from build123d import *

# Parameters (mm, degrees)
F0_W     = 13
F0_H     = 5
F1_DEPTH = 12
F2_W     = 11.2
F2_H     = 2
F3_DEPTH = 12
F4_W     = 9.4
F4_H     = 2
F5_DEPTH = 5.001
F7_DEPTH = 13
F8_W     = 1
F8_H     = 4
F9_DEPTH = 13.001


with BuildPart() as f1:
    # F0 (on Top) → F1 (new body)
    with BuildSketch(Plane.XY):
        Rectangle(F0_W, F0_H)
    extrude(amount=F1_DEPTH)

    # F2 (on face) → F3 (cut)
    with BuildSketch(Plane.XY.offset(12)):
        with Locations((0, 0.6)):
            Rectangle(F2_W, F2_H)
    extrude(amount=-F3_DEPTH, mode=Mode.SUBTRACT)

    # F4 (on face) → F5 (cut, through all)
    with BuildSketch(Plane(origin=(0, 2.5, 0), x_dir=(-1, 0, 0), z_dir=(0, 1, 0))):
        with Locations((0, 6)):
            Rectangle(F4_W, F4_H)
    extrude(amount=-F5_DEPTH, mode=Mode.SUBTRACT)

    # F6 (on face) → F7 (join)
    with BuildSketch(Plane(origin=(-6.5, 0, 0), x_dir=(0, -1, 0), z_dir=(-1, 0, 0))):
        with BuildLine():
            ThreePointArc((4.472136, -9.454356), (5.605034, -7.595289), (6, -5.454356))
            ThreePointArc((6, -5.454356), (5.049752, -2.213986), (2.5, 0))
            Line((2.5, 0), (-2.5, 0))
            ThreePointArc((-2.5, 0), (-5.873575, -4.229155), (-4.472136, -9.454356))
            ThreePointArc((-4.472136, -9.454356), (-1.428948, -1.652564), (5.25, -6.704356))
            ThreePointArc((5.25, -6.704356), (5.051792, -8.133304), (4.472136, -9.454356))
        make_face()
    extrude(amount=-F7_DEPTH)

    # F8 (on face) → F9 (cut, through all)
    with BuildSketch(Plane(origin=(-6.5, 0, 0), x_dir=(0, -1, 0), z_dir=(-1, 0, 0))):
        with Locations((0, 0.52178)):
            Rectangle(F8_W, F8_H)
    extrude(amount=-F9_DEPTH, mode=Mode.SUBTRACT)


solid = f1.part
Verification items for the finished model (mm, model axes). A direction names the side the tool comes from. Give positions to 0.01 mm unless a question says otherwise; leave off trailing zeros. Write each loop counter-clockwise with the first axis right and the second up, starting at its lowest first coordinate (ties: lowest second). Pieces come first, ordered by that corner, then holes. Notation, with made-up numbers: M 9,53 L 35,53 A26 cw 35,77 Z; hole C -38.75,62.25 d1. An arc over 180 degrees is marked long. Put each result on its own line as item: value. Start each with the question number.
1. Scan lines: line 1 along Y through (x, z) = (-5.5, 11.25); line 2 along X through (y, z) = (-0.5, 6.75); line 3 along X through (y, z) = (1.25, 5.25). Record each from-to range of solid material in increasing order. Write a range as [from, to].
2. Draft check along Z on faces 1 (the face through (5.6, 1, 6)), 2 (the face through (0, -1, 12)), 3 (the face through (0, -1, 5)). Enter one of: +Z half, -Z half, draft (parallel to the pull), parting line (faces both ways), or undercut.
3. Section check A-A (y = 0). Record the cut outline in (x, z).
4. Section check D-D (z = 8.75). Record the cut outline in (x, y), and give its area (3 significant figures).
5. Set-up check for faces 4 (the face through (-0.1, 0.5, -0.4)), 5 (the face through (-5.6, 1, 6)), 6 (the face through (-0.1, -0.4, 7.3)), 7 (the face through (4.7, 2, 6)), 8 (the face through (-0.09, 4.73, -4.43)): record each of +Z, -Z, +X, -X, +Y, -Y from which the full face is reachable in a straight line by a thin tool's end or side.
6. Go/stop test with flat-tipped pins: pin 1 Ø2 at (x, z) = (-0.5, -0.5) entering from -Y; pin 2 Ø5.5 at (x, z) = (-0.5, 4.5) entering from -Y; pin 3 Ø0.6 at (x, y) = (0.5, -1.5) entering from -Z. Record where each tip stops, or that it passes through.
7. Section check B-B (z = 6.5). Record the cut outline in (x, y).
8. Section check C-C (x = 2). Record the cut outline in (y, z), and give its area (3 significant figures).
Answer list:
1. line 1: [-2.5, -0.4], [1.6, 2.5]
1. line 2: [-6.5, -4.7], [4.7, 6.5]
1. line 3: [-6.5, -5.6], [5.6, 6.5]
2. face 1: draft
2. face 2: +Z half
2. face 3: undercut
3. outline: M -6.5,2.52 L -5.6,2.52 L -5.6,12 L -6.5,12 Z; M 5.6,2.52 L 6.5,2.52 L 6.5,12 L 5.6,12 Z
4. outline: M -6.5,-2.5 L 6.5,-2.5 L 6.5,2.5 L -6.5,2.5 Z; hole M -5.6,-0.4 L 5.6,-0.4 L 5.6,1.6 L -5.6,1.6 Z
4. area: 42.6 mm2
5. face 4: -Z, +X, -X
5. face 5: +Z
5. face 6: +Z, -Z
5. face 7: +Y, -Y
5. face 8: +X, -X
6. pin 1: y = -4.51
6. pin 2: y = -2.5
6. pin 3: z = -1.77
7. outline: M -6.5,-2.5 L -4.7,-2.5 L -4.7,-0.4 L -5.6,-0.4 L -5.6,1.6 L -4.7,1.6 L -4.7,2.5 L -6.5,2.5 Z; M 4.7,-2.5 L 6.5,-2.5 L 6.5,2.5 L 4.7,2.5 L 4.7,1.6 L 5.6,1.6 L 5.6,-0.4 L 4.7,-0.4 Z
8. outline: M -6,-5.45 A6 ccw -4.47,-9.45 A5.25 cw -5.25,-6.7 A5.25 cw -0.5,-1.48 L -0.5,2.52 L -0.4,2.52 L -0.4,5 L -2.5,5 L -2.5,0 A6 ccw Z; M -2.5,7 L -0.4,7 L -0.4,12 L -2.5,12 Z; M 0.5,-1.48 A5.25 cw 4.47,-9.45 A6 ccw 2.5,0 L 2.5,5 L 1.6,5 L 1.6,0 L 0.5,0 Z; M 1.6,7 L 2.5,7 L 2.5,12 L 1.6,12 Z
8. area: 56.4 mm2
